from build123d import *

# Parameters (mm, degrees)
F0_W     = 37
F0_H     = 30
F1_DEPTH = 12
F2_R     = 7
F3_DEPTH = 10
F4_R     = 2
F5_DEPTH = 8
F6_R     = 2
F7_DEPTH = 8
F8_R     = 6
F9_DEPTH = 25


with BuildPart() as f1:
    # F0 (on Top) → F1 (new body)
    with BuildSketch(Plane.XY):
        with Locations((18.5, -15)):
            Rectangle(F0_W, F0_H)
    extrude(amount=F1_DEPTH)

    # F2 (on face) → F3 (cut)
    with BuildSketch(Plane.XY.offset(12)):
        with Locations((18.5, -15)):
            Circle(F2_R)
    extrude(amount=-F3_DEPTH, mode=Mode.SUBTRACT)

    # F4 (on face) → F5 (cut)
    with BuildSketch(Plane.YZ.offset(37)):
        with Locations((-5, 6)):
            Circle(F4_R)
        with Locations((-25, 6)):
            Circle(F4_R)
    extrude(amount=-F5_DEPTH, mode=Mode.SUBTRACT)

    # F6 (on face) → F7 (cut)
    with BuildSketch(Plane(origin=(0, 0, 0), x_dir=(0, -1, 0), z_dir=(-1, 0, 0))):
        with Locations((25, 6)):
            Circle(F6_R)
        with Locations((5, 6)):
            Circle(F6_R)
    extrude(amount=-F7_DEPTH, mode=Mode.SUBTRACT)

    # F8 (on face) → F9 (cut)
    with BuildSketch(Plane.XY.offset(2)):
        with Locations((18.5, -15)):
            Circle(F8_R)
    extrude(amount=-F9_DEPTH, mode=Mode.SUBTRACT)


solid = f1.part
Check sheet for the modelled part. Datum: model origin and axes. Units: mm. A direction names the side the tool comes from. Give positions to 0.01 mm unless a question says otherwise; leave off trailing zeros. Write each loop counter-clockwise with the first axis right and the second up, starting at its lowest first coordinate (ties: lowest second). Pieces come first, ordered by that corner, then holes. Notation, with made-up numbers: (46, -40) -> (73, -40) arc R21 ccw to (73, -17) -> close; hole circle Ø3 at (2, 41). An arc over 180 degrees is marked (long way). Write item = value, one per line.
Item 1: Sectioned sample at D-D on x = 18.5. Record the boundary of the cut face in (y, z), and give its area (3 significant figures).
Output:
outline = (-30, 0) -> (-21, 0) -> (-21, 2) -> (-22, 2) -> (-22, 12) -> (-30, 12) -> close; (-9, 0) -> (0, 0) -> (0, 12) -> (-8, 12) -> (-8, 2) -> (-9, 2) -> close
area = 196 mm^2
Item 2: Sectioned sample at B-B on x = 30. Record the boundary of the cut face in (y, z), and give its area (3 significant figures).
Output:
outline = (-30, 0) -> (0, 0) -> (0, 12) -> (-30, 12) -> close; hole circle Ø4 at (-25, 6); hole circle Ø4 at (-5, 6)
area = 335 mm^2
Item 3: Scan lines: probe 1 along X at (y, z) = (-15.25, 7.75); probe 2 along Y at (x, z) = (18.5, 0.75); probe 3 along Y at (x, z) = (18.5, 9.5). Record each from-to range of solid material in increasing order. Write a range as from..to.
Output:
probe_1 = 0..11.5, 25.5..37
probe_2 = -30..-21, -9..0
probe_3 = -30..-22, -8..0
Item 4: Gauge pin test, flat ends, axial feed: pin 1 (3 mm diameter, centred on y = -5, z = 6, fed in from +X); pin 2 (1.2 mm diameter, centred on y = -25.5, z = 5, fed in from -X); pin 3 (4 mm diameter, centred on x = 29.5, y = -10.5, fed in from -Z); pin 4 (4 mm diameter, centred on x = 21, y = -15, fed in from +Z) (1 decimal). Record the tip position at first contact, or that the pin passes through.
Output:
pin_1 = 29
pin_2 = 8
pin_3 = 0
pin_4 = through
Item 5: Release check for a two-part mould opening along Y. For faces 1 (the cylindrical face through (33, -27, 6)), 2 (the flat face through (0, -15, 6)), 3 (the flat face through (18, 0, 6)) record: +Y half, -Y half, draft (parallel to the pull), parting line (faces both ways), or undercut.
Output:
face_1 = undercut
face_2 = draft
face_3 = +Y half
Item 6: Tool access check on faces 4 (the flat face through (29, -5, 6)), 5 (the cylindrical face through (11.507, -14.692, 7.07)), 6 (the cylindrical face through (4, -23, 6)). Record the directions out of +Z, -Z, +X, -X, +Y, -Y that give a thin tool (end or side, any length) a straight path to the whole face; none if there is none.
Output:
face_4 = +X
face_5 = +Z
face_6 = -X
Item 7: Sectioned sample at C-C on z = 3. Record the boundary of the cut face in (x, y).
Output:
outline = (0, -30) -> (37, -30) -> (37, 0) -> (0, 0) -> close; hole circle Ø14 at (18.5, -15)
Item 8: Sectioned sample at A-A on y = -15. Record the boundary of the cut face in (x, z).
Output:
outline = (0, 0) -> (12.5, 0) -> (12.5, 2) -> (11.5, 2) -> (11.5, 12) -> (0, 12) -> close; (24.5, 0) -> (37, 0) -> (37, 12) -> (25.5, 12) -> (25.5, 2) -> (24.5, 2) -> close
